Geometry: final body of the model. Coordinates: model frame, mm. Face numbers are marked on the shaded views. A direction names the side the tool comes from. Round coordinates to 2 decimals unless told otherwise and drop trailing zeros. Loops run counter-clockwise (first coordinate to the right, second up) from the corner with the lowest first, then second, coordinate; pieces in that order, holes last. Notation, with made-up numbers: (2, 4) -> (60, 4) arc R5 ccw to (60, 12) -> close; hole circle Ø4 at (57.25, 20.5). An arc over 180 degrees is marked (long way). Answer in a Markdown table with one row per item.
```python
from build123d import *

# Parameters (mm, degrees)
F0_R            = 22
F1_DEPTH        = 82
F2_T            = -1.95
F0_R_2          = 28
F3_DEPTH        = 3
F5_R            = 5.05
F6_DEPTH        = 90
F7_R            = 1.55
F8_DEPTH        = 5
F8_COPIES_COUNT = 18
F10_R           = 11
F12_R           = 9.5
F13_DEPTH       = 30
F15_W           = 40
F15_H           = 3
F17_R           = 6
F18_DEPTH       = 10
F19_R           = 5


# Not quite as in the source:
# - a pattern or mirror of a feature is missing from the dataset's text; its kind, count and spacing are read off the source's solid


with BuildPart() as f1:
    # F0 (on Top) → F1 (new body)
    with BuildSketch(Plane.XY):
        Circle(F0_R)
    extrude(amount=F1_DEPTH)

    # F2
    f2_openings = [f1.faces().sort_by_distance(p)[0] for p in [
        (0, 0, 0),
    ]]
    offset(amount=F2_T, openings=f2_openings)

    # F0 (on Top) → F3 (join)
    with BuildSketch(Plane.XY):
        Circle(F0_R_2)
        Circle(F0_R, mode=Mode.SUBTRACT)
    extrude(amount=F3_DEPTH)

    # F5 (on Top) → F6 (cut)
    with BuildSketch(Plane.XY):
        Circle(F5_R)
    extrude(amount=F6_DEPTH, mode=Mode.SUBTRACT)

    # F7 (on face) → F8 (cut)
    with BuildSketch(Plane.XY):
        with Locations((-5.3322692402, -24.1057705134)):
            Circle(F7_R)
    f8 = extrude(amount=F8_DEPTH, mode=Mode.SUBTRACT)

    # F8_copies: F8 ×18 about axis
    f8_copies_axis = Axis((0, 0, 0), (0, 0, 1))
    for i in range(1, F8_COPIES_COUNT):
        add(f8.rotate(f8_copies_axis, i * 360 / F8_COPIES_COUNT), mode=Mode.SUBTRACT)

    # F10 (on offset) → F11 (join, up to the next surface of F1)
    with BuildSketch(Plane.XZ.offset(40)):
        with Locations((0, 64.2171450533)):
            Circle(F10_R)
    extrude(until=Until.NEXT, dir=(0, 1, 0))

    # F12 (on face) → F13 (cut)
    with BuildSketch(Plane.XZ.offset(40)):
        with Locations((0, 64.2171450533)):
            Circle(F12_R)
    extrude(amount=-F13_DEPTH, mode=Mode.SUBTRACT)

    # F15 (on offset) → F16 (join, up to the next surface of F1)
    with BuildSketch(Plane.XZ.offset(-60)):
        with Locations((-0.2395864576, 76.434844184)):
            Rectangle(F15_W, F15_H)
    extrude(until=Until.NEXT)

    # F17 (on face) → F18 (cut)
    with BuildSketch(Plane.XY.offset(82)):
        with BuildLine():
            Line((15.5, 56.001), (15.5, 54.501))
            ThreePointArc((15.5, 54.501), (16.5606601718, 54.9403398282), (17, 56.001))
            ThreePointArc((17, 56.001), (15.5, 57.501), (14, 56.001))
            Line((14, 56.001), (15.5, 56.001))
        make_face()
        with BuildLine():
            ThreePointArc((14, 56.001), (14.4393398282, 54.9403398282), (15.5, 54.501))
            Line((15.5, 54.501), (15.5, 56.001))
            Line((15.5, 56.001), (14, 56.001))
        make_face()
        with BuildLine():
            ThreePointArc((-14, 56.001), (-16.5606601718, 57.0616601718), (-15.5, 54.501))
            Line((-15.5, 54.501), (-15.5, 56.001))
            Line((-15.5, 56.001), (-14, 56.001))
        make_face()
        with BuildLine():
            Line((-15.5, 56.001), (-15.5, 54.501))
            ThreePointArc((-15.5, 54.501), (-14.4393398282, 54.9403398282), (-14, 56.001))
            Line((-14, 56.001), (-15.5, 56.001))
        make_face()
        with BuildLine():
            ThreePointArc((-15.5, 26.501), (-16.5606601718, 23.9403398282), (-14, 25.001))
            Line((-14, 25.001), (-15.5, 25.001))
            Line((-15.5, 25.001), (-15.5, 26.501))
        make_face()
        with BuildLine():
            Line((-15.5, 25.001), (-14, 25.001))
            ThreePointArc((-14, 25.001), (-14.4393398282, 26.0616601718), (-15.5, 26.501))
            Line((-15.5, 26.501), (-15.5, 25.001))
        make_face()
        with BuildLine():
            Line((15.5, 25.001), (14, 25.001))
            ThreePointArc((14, 25.001), (15.5, 23.501), (17, 25.001))
            ThreePointArc((17, 25.001), (16.5606601718, 26.0616601718), (15.5, 26.501))
            Line((15.5, 26.501), (15.5, 25.001))
        make_face()
        with BuildLine():
            ThreePointArc((15.5, 26.501), (14.4393398282, 26.0616601718), (14, 25.001))
            Line((14, 25.001), (15.5, 25.001))
            Line((15.5, 25.001), (15.5, 26.501))
        make_face()
        with Locations((0, 40.501)):
            Circle(F17_R)
    extrude(amount=-F18_DEPTH, mode=Mode.SUBTRACT)

    # F19
    f19_edges = [f1.edges().sort_by_distance(p)[0] for p in [
        (-20.239586, 60, 76.434844),
        (19.760414, 60, 76.434844),
    ]]
    fillet(f19_edges, radius=F19_R)


solid = f1.part
```
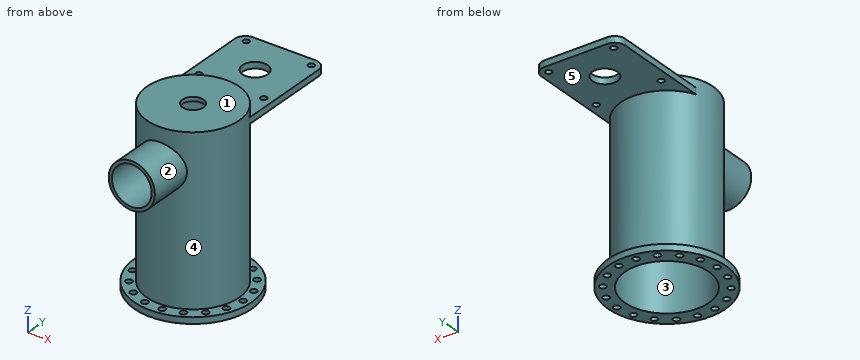
Item 1: Set-up query: the marked faces 1 and 2. Return all of +Z, -Z, +X, -X, +Y, -Y with unobstructed straight access to the full face (end or side cutting, diameter ignored); none if empty.
Ans:
| item | result |
|---|---|
| face 1 | +Z, +X, -X, +Y, -Y |
| face 2 | -Y |
Item 2: Section query C-C, the plane z = 59. Output: boundary loops of the cut face in (x, y), and give its area (3 significant figures).
Ans:
| item | result |
|---|---|
| outline | (-9.68, -40) -> (-7.94, -40) -> (-7.94, -18.41) arc R20.05 cw (long way) to (7.94, -18.41) -> (7.94, -40) -> (9.68, -40) -> (9.68, -19.75) arc R22 ccw (long way) to (-9.68, -19.75) -> close |
| area | 295 mm2 |
Item 3: Mould query, pull axis X, two halves, no side actions, for the marked faces 3, 4 and 5. Classes: released by +X, released by -X, zero draft, split by the parting line, or undercut.
Ans:
| item | result |
|---|---|
| face 3 | undercut |
| face 4 | split by the parting line |
| face 5 | zero draft |
Item 4: Section query B-B, the plane z = 33. Output: boundary loops of the cut face in (x, y).
Ans:
| item | result |
|---|---|
| outline | circle Ø44 at (0, 0); hole circle Ø40.1 at (0, 0) |
Item 5: Ray query, L1, parallel to Z at x = -5, y = 26; L2, parallel to X at y = 0.5, z = 44.5; L3, parallel to Y at x = 0, z = 47. Return the intervals inside material, ascending.
Ans:
| item | result |
|---|---|
| L1 | 0 to 3, 74.93 to 77.93 |
| L2 | -21.99 to -20.04, 20.04 to 21.99 |
| L3 | -22 to -20.05, 20.05 to 22 |
Item 6: First-contact query: P1, Ø1.5, axis at y = 5.5, z = 10.5, coming from the -X side; P2, Ø4, axis at x = -11.41, y = 21.89, coming from the +Z side; P3, Ø2.5, axis at x = 5.33, y = 24.11, coming from the -Z side. Flat tips, straight axial feed; report the tip coordinate or a pass-through.
Ans:
| item | result |
|---|---|
| P1 | x = -21.48 |
| P2 | z = 77.93 |
| P3 | z = 74.93 |
Item 7: Section query A-A, the plane x = 0. State how many separate pieces and enclosed holes the cut face has, and give its area (3 significant figures).
Ans:
| item | result |
|---|---|
| separate pieces | 4 |
| enclosed holes | 0 |
| area | 509 mm2 |
